Geometry check sheet. Reference: the model listing, model coordinates, mm. Give positions to 0.01 mm unless a question says otherwise; leave off trailing zeros. Order: outer loops, then holes, each group sorted by start corner. A loop starts at its lowest first (then second) coordinate and runs counter-clockwise, first axis right, second up.
from build123d import *

# Parameters (mm, degrees)
ESQUISSE1_W                  = 90
ESQUISSE1_H                  = 98
BOSS_EXTRU_1_DEPTH           = 1
ENL_V_MAT_EXTRU_1_DEPTH      = 134.06013678
ENL_V_MAT_EXTRU_1_DEPTH_BACK = 134.06013678
ESQUISSE2_R                  = 1.6


with BuildPart() as part:
    # Esquisse1 → Boss.-Extru.1 (new body)
    with BuildSketch(Plane.XY):
        with Locations((45, 49)):
            Rectangle(ESQUISSE1_W, ESQUISSE1_H)
    extrude(amount=BOSS_EXTRU_1_DEPTH)

    # Esquisse2 → Enlèv. mat.-Extru.1 (cut, two sides: drawn at the far end of the back side and taken through both)
    with BuildSketch(Plane.XY.offset(1).offset(-ENL_V_MAT_EXTRU_1_DEPTH_BACK)):
        with Locations((7, 50)):
            Circle(ESQUISSE2_R)
        with Locations((7, 90)):
            Circle(ESQUISSE2_R)
        with Locations(Location((83, 90, 0), (0, 0, 180))):
            Circle(ESQUISSE2_R)
        with Locations(Location((83, 50, 0), (0, 0, 180))):
            Circle(ESQUISSE2_R)
    extrude(amount=ENL_V_MAT_EXTRU_1_DEPTH + ENL_V_MAT_EXTRU_1_DEPTH_BACK, mode=Mode.SUBTRACT)


solid = part.part
Item 1: Sectioned sample at A-A (x = 83). Enter the section's corners in (y, z), and give its area (3 significant figures).
Reported:
outline: (0, 0) - (48.4, 0) - (48.4, 1) - (0, 1) - close; (51.6, 0) - (88.4, 0) - (88.4, 1) - (51.6, 1) - close; (91.6, 0) - (98, 0) - (98, 1) - (91.6, 1) - close
area: 91.6 mm2
Item 2: Draft check along Y on faces 1 (the flat face through (44, 50, 1)), 2 (the cylindrical face through (81.474, 89.519, 0.493)). Enter one of: released by +Y, released by -Y, zero draft, split by the parting line, or undercut.
Reported:
face 1: zero draft
face 2: undercut
Item 3: Sectioned sample at B-B (y = 50). Enter the section's corners in (x, z), and give its area (3 significant figures).
Reported:
outline: (0, 0) - (5.4, 0) - (5.4, 1) - (0, 1) - close; (8.6, 0) - (81.4, 0) - (81.4, 1) - (8.6, 1) - close; (84.6, 0) - (90, 0) - (90, 1) - (84.6, 1) - close
area: 83.6 mm2
Item 4: Scan lines: L1, parallel to Y at x = 83, z = 0.85; L2, parallel to X at y = 90, z = 0.85; L3, parallel to X at y = 91, z = 0.15. Record each from-to range of solid material in increasing order.
Reported:
L1: y = 0 to 48.4, 51.6 to 88.4, 91.6 to 98
L2: x = 0 to 5.4, 8.6 to 81.4, 84.6 to 90
L3: x = 0 to 5.75, 8.25 to 81.75, 84.25 to 90
